```python
from build123d import *

# Parameters (mm, degrees)
F0_W     = 190
F0_H     = 270
F0_R     = 2.5
F0_R_2   = 80
F0_R_3   = 2.6
F1_DEPTH = 3.2


# Not quite as in the source:
# - a feature names something its author has since deleted; it is built from what else it names


with BuildPart() as f1:
    # F0 (on Top) → F1 (new body)
    with BuildSketch(Plane.XY):
        Rectangle(F0_W, F0_H)
        with Locations((-85, -125)):
            Circle(F0_R, mode=Mode.SUBTRACT)
        with Locations((85, -125)):
            Circle(F0_R, mode=Mode.SUBTRACT)
        with Locations((-85, 125)):
            Circle(F0_R, mode=Mode.SUBTRACT)
        with Locations((0, 40)):
            Circle(F0_R_2, mode=Mode.SUBTRACT)
        with Locations((85, 125)):
            Circle(F0_R, mode=Mode.SUBTRACT)
        with Locations((0, 40)):
            Circle(F0_R_2)
        with Locations((0, 40)):
            Circle(F0_R_3, mode=Mode.SUBTRACT)
    extrude(amount=F1_DEPTH)


solid = f1.part
```
Work out the finished part from the listing and answer in its coordinate system (mm). Round coordinates to 2 decimals unless told otherwise and drop trailing zeros.
1) Consider probe 1 along Y at (x, z) = (-85, 1.05); probe 2 along Y at (x, z) = (0, 1.3). Determine where each line is inside the solid, lowest interval first.
2) A flat-ended cylindrical pin translates along its axis: P1, Ø5, axis at x = 51, y = 98, coming from the -Z side. Find the tip coordinate at first contact, or state that the pin passes through.
3) Determine the mould class of faces 1 (the face through (-85.33, 127.48, 1.58)), 2 (the face through (-1, 2, 0)) for opening direction X: pulls with the +X half, pulls with the -X half, needs draft (parallel to the pull), parting line crosses it, or undercut.
Entries:
1. probe 1: y = -135 to -127.5, -122.5 to 122.5, 127.5 to 135
1. probe 2: y = -135 to 37.4, 42.6 to 135
2. P1: stops at z = 0
3. face 1: undercut
3. face 2: needs draft
